Geometry: final body of the model. Coordinates: model frame, mm. Face numbers are marked on the shaded views. A direction names the side the tool comes from. Round coordinates to 2 decimals unless told otherwise and drop trailing zeros. Loops run counter-clockwise (first coordinate to the right, second up) from the corner with the lowest first, then second, coordinate; pieces in that order, holes last. Notation, with made-up numbers: (78, 72.25) - (134, 72.25) arc R20 cw to (134, 97.25) - close; hole circle Ø5 at (-19, -24). An arc over 180 degrees is marked (long way). Answer as a JSON object with one key per item and string values. Group by question number.
Item 1: Line query: line 1 (X direction, y = 5.25, z = 12.75); line 2 (Y direction, x = 0, z = 0.85); line 3 (Z direction, x = -4, y = 5). Output: solid intervals per line, ascending.
Item 2: Reachability of the marked faces 1 and 2 from +Z, -Z, +X, -X, +Y, -Y: full face, straight path, thin tool, end or side. Return the list, or none.
Item 3: Section D-D (z = 15). Return the cut outline in (x, y).
Item 4: Section C-C (y = -2.25). Return the cut outline in (x, z), plus the area to 3 significant figures.
Item 5: Section B-B (z = 17.5). Return the cut outline in (x, y).
Item 6: First-contact query: pin 1 (4 mm diameter, centred on y = 0.51, z = 13.74, fed in from -X); pin 2 (1.5 mm diameter, centred on x = -2.5, y = 3.5, fed in from +Z). Flat tips, straight axial feed; report the tip coordinate or a pass-through.
Item 7: Section A-A (x = -1.5). Return the cut outline in (y, z), plus the area to 3 significant figures.
Item 8: Draft query along Z for the marked faces 3, 4 and 5. Return one class per face: released by +Z, released by -Z, zero draft, split by the parting line, or undercut.
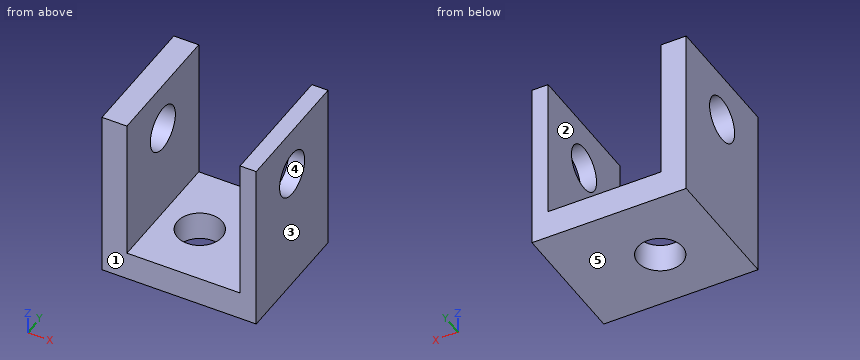
```python
from build123d import *

# Parameters (mm, degrees)
SKETCH1_W           = 17.180000002
SKETCH1_H           = 14.347137423
SKETCH1_R           = 2.5
BOSS_EXTRUDE1_DEPTH = 3.18
SKETCH2_W           = 1.798380988
SKETCH2_H           = 14.347137423
SKETCH2_W_2         = 2.781619014
BOSS_EXTRUDE2_DEPTH = 15.932476
SKETCH3_R           = 2.5
CUT_EXTRUDE1_DEPTH  = 27.822965215


with BuildPart() as part:
    # Sketch1 → Boss-Extrude1 (new body)
    with BuildSketch(Plane.XY):
        with Locations((1.409999999, 0.509680861)):
            Rectangle(SKETCH1_W, SKETCH1_H)
        with Locations(Location((0, 0, 0), (0, 0, 180))):
            Circle(SKETCH1_R, mode=Mode.SUBTRACT)
    extrude(amount=BOSS_EXTRUDE1_DEPTH)

    # Sketch2 → Boss-Extrude2 (add)
    with BuildSketch(Plane.XY.offset(3.18)):
        with Locations((9.100809506, 0.509680861)):
            Rectangle(SKETCH2_W, SKETCH2_H)
        with Locations((-5.789190495, 0.509680861)):
            Rectangle(SKETCH2_W_2, SKETCH2_H)
    extrude(amount=BOSS_EXTRUDE2_DEPTH)

    # Sketch3 → Cut-Extrude1 (cut, through all)
    with BuildSketch(Plane(origin=(10, 0, 0), x_dir=(0, 0, -1), z_dir=(1, 0, 0))):
        with Locations(Location((-13.737500001, 0.50968086, 0), (0, 0, 90))):
            Circle(SKETCH3_R)
    extrude(amount=-CUT_EXTRUDE1_DEPTH, mode=Mode.SUBTRACT)


solid = part.part
```
Values:
{
 "1": {"line 1": "x = -7.18 to -4.4, 8.2 to 10", "line 2": "y = -6.66 to -2.5, 2.5 to 7.68", "line 3": "z = 0 to 3.18"},
 "2": {"face 1": "+Z, -Z, +X, -X, -Y", "face 2": "+Z, +Y, -Y"},
 "3": {"outline": "(-7.18, -6.66) - (-4.4, -6.66) - (-4.4, -1.65) - (-7.18, -1.65) - close; (-7.18, 2.67) - (-4.4, 2.67) - (-4.4, 7.68) - (-7.18, 7.68) - close; (8.2, -6.66) - (10, -6.66) - (10, -1.65) - (8.2, -1.65) - close; (8.2, 2.67) - (10, 2.67) - (10, 7.68) - (8.2, 7.68) - close"},
 "4": {"outline": "(-7.18, 0) - (-1.09, 0) - (-1.09, 3.18) - (-4.4, 3.18) - (-4.4, 19.11) - (-7.18, 19.11) - close; (1.09, 0) - (10, 0) - (10, 19.11) - (8.2, 19.11) - (8.2, 3.18) - (1.09, 3.18) - close", "area": "121 mm^2"},
 "5": {"outline": "(-7.18, -6.66) - (-4.4, -6.66) - (-4.4, 7.68) - (-7.18, 7.68) - close; (8.2, -6.66) - (10, -6.66) - (10, 7.68) - (8.2, 7.68) - close"},
 "6": {"pin 1": "passes through", "pin 2": "stops at z = 3.18"},
 "7": {"outline": "(-6.66, 0) - (-2, 0) - (-2, 3.18) - (-6.66, 3.18) - close; (2, 0) - (7.68, 0) - (7.68, 3.18) - (2, 3.18) - close", "area": "32.9 mm^2"},
 "8": {"face 3": "zero draft", "face 4": "undercut", "face 5": "released by -Z"}
}
